Check sheet for the modelled part. Datum: model origin and axes. Units: mm. A direction names the side the tool comes from. Coordinates: 2 decimals unless noted, no trailing zeros. Order: outer loops, then holes, each group sorted by start corner. A loop starts at its lowest first (then second) coordinate and runs counter-clockwise, first axis right, second up.
from build123d import *
from OCP.BRepFilletAPI import BRepFilletAPI_MakeChamfer

# Parameters (mm, degrees)
CROQUIS1_W              = 66
CROQUIS1_H              = 110
SALIENTE_EXTRUIR1_DEPTH = 3
SALIENTE_EXTRUIR2_DEPTH = 28
CROQUIS3_W              = 107
CROQUIS3_H              = 2
SALIENTE_EXTRUIR3_DEPTH = 2
REDONDEO1_R             = 5
CHAFL_N1_SIZE           = 3
CHAFL_N1_SIZE2          = 1.091910703
CHAFL_N2_START          = -54
CHAFL_N2_OUTLINE_W      = 7
CHAFL_N2_OUTLINE_H      = 9
CHAFL_N2_DEPTH          = 3.770526581
CHAFL_N3_START          = 50.229473419
CHAFL_N3_OUTLINE_W      = 8
CHAFL_N3_OUTLINE_H      = 9
CHAFL_N3_DEPTH          = 3.770526581


with BuildPart() as part:
    # Croquis1 → Saliente-Extruir1 (new body)
    with BuildSketch(Plane(origin=(0, 0, 0), x_dir=(1, 0, 0), z_dir=(0, 1, 0))):
        Rectangle(CROQUIS1_W, CROQUIS1_H)
    extrude(amount=SALIENTE_EXTRUIR1_DEPTH)

    # Croquis2 → Saliente-Extruir2 (add)
    with BuildSketch(Plane.XZ):
        Polygon((-28, 55), (-33, 55), (-33, -49.5), (-33, -55), (-28, -55), (28, -55), (33, -55), (33, -52), (33, 55), (28, 55), (28, -52), (-28, -52), align=None)
    extrude(amount=SALIENTE_EXTRUIR2_DEPTH)

    # Croquis3 → Saliente-Extruir3 (add)
    with BuildSketch(Plane(origin=(-28, 0, 0), x_dir=(0, 0, -1), z_dir=(1, 0, 0))):
        with Locations((-1.5, -21)):
            Rectangle(CROQUIS3_W, CROQUIS3_H)
    saliente_extruir3 = extrude(amount=SALIENTE_EXTRUIR3_DEPTH)

    # Simetría1: Saliente-Extruir3 across plane
    add(saliente_extruir3.mirror(Plane(origin=(0, 0, 0), x_dir=(0, 0, 1), z_dir=(1, 0, 0))))

    # Redondeo1
    redondeo1_edges = [part.edges().sort_by_distance(p)[0] for p in [
        (-33, -12.5, -55),
        (33, -12.5, -55),
    ]]
    fillet(redondeo1_edges, radius=REDONDEO1_R)

    # Chaflán1: one chamfer whose edges measure the first distance from different faces: ONE call of the kernel's chamfer builder (chamfer() names one face for all edges)
    chafl_n1_edges_1 = [part.edges().sort_by_distance(p)[0] for p in [
        (-33, -28, 2.5),
    ]]
    chafl_n1_side_1 = [part.faces().sort_by_distance(p)[0] for p in [
        (-33, -12.5, 2.5),
    ]]
    chafl_n1_edges_2 = [part.edges().sort_by_distance(p)[0] for p in [
        (0, -28, -55),
    ]]
    chafl_n1_side_2 = [part.faces().sort_by_distance(p)[0] for p in [
        (0, -12.5, -55),
    ]]
    chafl_n1_edges_3 = [part.edges().sort_by_distance(p)[0] for p in [
        (33, -28, 2.5),
    ]]
    chafl_n1_side_3 = [part.faces().sort_by_distance(p)[0] for p in [
        (33, -12.5, 2.5),
    ]]
    chafl_n1_edges_4 = [part.edges().sort_by_distance(p)[0] for p in [
        (31.535533906, -28, -53.535533906),
    ]]
    chafl_n1_side_4 = [part.faces().sort_by_distance(p)[0] for p in [
        (31.535533906, -12.5, -53.535533906),
    ]]
    chafl_n1_edges_5 = [part.edges().sort_by_distance(p)[0] for p in [
        (-31.535533906, -28, -53.535533906),
    ]]
    chafl_n1_side_5 = [part.faces().sort_by_distance(p)[0] for p in [
        (-31.535533906, -12.5, -53.535533906),
    ]]
    chafl_n1 = BRepFilletAPI_MakeChamfer(part.part.solid().wrapped)
    for e in chafl_n1_edges_1:
        chafl_n1.Add(CHAFL_N1_SIZE, CHAFL_N1_SIZE2, e.wrapped, chafl_n1_side_1[0].wrapped)  # the first distance lies on this face
    for e in chafl_n1_edges_2:
        chafl_n1.Add(CHAFL_N1_SIZE, CHAFL_N1_SIZE2, e.wrapped, chafl_n1_side_2[0].wrapped)  # the first distance lies on this face
    for e in chafl_n1_edges_3:
        chafl_n1.Add(CHAFL_N1_SIZE, CHAFL_N1_SIZE2, e.wrapped, chafl_n1_side_3[0].wrapped)  # the first distance lies on this face
    for e in chafl_n1_edges_4:
        chafl_n1.Add(CHAFL_N1_SIZE, CHAFL_N1_SIZE2, e.wrapped, chafl_n1_side_4[0].wrapped)  # the first distance lies on this face
    for e in chafl_n1_edges_5:
        chafl_n1.Add(CHAFL_N1_SIZE, CHAFL_N1_SIZE2, e.wrapped, chafl_n1_side_5[0].wrapped)  # the first distance lies on this face
    add(Compound.cast(chafl_n1.Shape()), mode=Mode.REPLACE)

    # Chaflán2: read off the stored shape, not the designer's step
    # Chaflán2 outline → Chaflán2 (cut)
    with BuildSketch(Plane(origin=(0, 0, 0), x_dir=(0.8164965809277258, 0.40824829046386313, 0.40824829046386313), z_dir=(0.5773502691896258, -0.5773502691896258, -0.5773502691896258)).offset(CHAFL_N2_START)):
        with Locations((-2.5, 36.5)):
            Rectangle(CHAFL_N2_OUTLINE_W, CHAFL_N2_OUTLINE_H)
    extrude(amount=CHAFL_N2_DEPTH, mode=Mode.SUBTRACT)

    # Chaflán3: read off the stored shape, not the designer's step
    # Chaflán3 outline → Chaflán3 (cut)
    with BuildSketch(Plane(origin=(0, 0, 0), x_dir=(0.8164965809277258, -0.40824829046386313, -0.40824829046386313), z_dir=(0.5773502691896258, 0.5773502691896258, 0.5773502691896258)).offset(CHAFL_N3_START)):
        with Locations((2, -36.5)):
            Rectangle(CHAFL_N3_OUTLINE_W, CHAFL_N3_OUTLINE_H)
    extrude(amount=CHAFL_N3_DEPTH, mode=Mode.SUBTRACT)


solid = part.part
(1) Cross-section at A-A (x = -11). Enter the section's corners in (y, z), and give its area (3 significant figures).
Filled in:
outline: (-28, -53.91) - (-25, -55) - (3, -55) - (3, 55) - (0, 55) - (0, -52) - (-28, -52) - close
area: 412 mm2
(2) Cross-section at C-C (z = -46.5). Enter the section's corners in (x, y).
Filled in:
outline: (-33, -25) - (-31.91, -28) - (-28, -28) - (-28, -22) - (-26, -22) - (-26, -20) - (-28, -20) - (-28, 0) - (28, 0) - (28, -20) - (26, -20) - (26, -22) - (28, -22) - (28, -28) - (31.91, -28) - (33, -25) - (33, 3) - (-33, 3) - close
(3) Thickness scan on probe 1 along X at (y, z) = (-4.5, -49); probe 2 along Y at (x, z) = (26.5, -37.5); probe 3 along Z at (x, y) = (-10.5, -1.5). Record the ranges inside material, lowest first.
Filled in:
probe 1: x = -33 to -28, 28 to 33
probe 2: y = -22 to -20, 0 to 3
probe 3: z = -55 to -52
(4) Cross-section at B-B (y = -3.5). Enter the section's corners in (x, z), and give its area (3 significant figures).
Filled in:
outline: (-33, -50) arc R5 ccw to (-28, -55) - (28, -55) arc R5 ccw to (33, -50) - (33, 55) - (28, 55) - (28, -52) - (-28, -52) - (-28, 55) - (-33, 55) - close
area: 1,260 mm2
(5) Release check for a two-part mould opening along X. For faces 4 (the flat face through (-0.392, -26.521, -54.446)), 5 (the flat face through (32.446, -26.521, 1.765)), 6 (the flat face through (28, -10, 2)) record: +X half, -X half, draft (parallel to the pull), parting line (faces both ways), or undercut.
Filled in:
face 4: draft
face 5: +X half
face 6: undercut
(6) Tool access check on faces 1 (the flat face through (-26, -21, 2)), 2 (the flat face through (-29, -28, 1)), 3 (the flat face through (-28, -10, 1)). Record the directions out of +Z, -Z, +X, -X, +Y, -Y that give a thin tool (end or side, any length) a straight path to the whole face; none if there is none.
Filled in:
face 1: +Z, -Y
face 2: +Z, -Z, +X, -X, -Y
face 3: +Z
(7) Go/stop test with flat-tipped pins: P1, Ø8.5, axis at x = 8, y = -13.5, coming from the +Z side; P2, Ø1, axis at x = 27, z = -3, coming from the -Y side; P3, Ø17, axis at x = 8.5, z = -17.5, coming from the -Y side. Record where each tip stops, or that it passes through.
Filled in:
P1: stops at z = -52
P2: stops at y = -22
P3: stops at y = 0
